Part model, mm, in its own coordinate system. Face numbers are marked on the shaded views. Give positions to 0.01 mm unless a question says otherwise; leave off trailing zeros. Order: outer loops, then holes, each group sorted by start corner. A loop starts at its lowest first (then second) coordinate and runs counter-clockwise, first axis right, second up. Notation, with made-up numbers: (12.25, 30) -> (70.25, 30) arc R22 cw to (70.25, 63) -> close; hole circle Ø5 at (65.25, -29.5). An arc over 180 degrees is marked (long way). Write item = value, one per line. Start each with the question number.
Item 1: Flat gauge pins, fed straight in: P1, Ø23, axis at x = 4, z = -10.5, coming from the -Y side; P2, Ø2, axis at x = 5.5, y = 14, coming from the +Z side; P3, Ø1, axis at y = 31, z = -0.5, coming from the -X side; P4, Ø8, axis at y = 11, z = -18, coming from the -X side. Where does each tip first touch, or does it go through?
Item 2: Band-saw the part on B-B on z = -17.5. Write the cut outline in (x, y).
Item 3: Band-saw the part on C-C on z = 20. Write the cut outline in (x, y).
Item 4: Drill centre lines: line 1 along Y through (x, z) = (1.5, -2); line 2 along X through (y, z) = (3, -0.5); line 3 along X through (y, z) = (29, 21). Where is each one in solid material? Low to high.
Item 5: Band-saw the part on A-A on y = 5. Write the cut outline in (x, z), plus the area to 3 significant figures.
Item 6: Pull direction X, two halves, no side cores. Call the marked faces 1, 2 and 3: +X half, -X half, draft (parallel to the pull), parting line (faces both ways), or undercut.
```python
from build123d import *

# Parameters (mm, degrees)
SKETCH1_R           = 22.86
BOSS_EXTRUDE1_DEPTH = 43.18
SKETCH3_R           = 3.81
BOSS_EXTRUDE2_DEPTH = 2.54
BOSS_EXTRUDE2_TAPER = 52
CIRPATTERN1_COUNT   = 8


with BuildPart() as part:
    # Sketch1 → Boss-Extrude1 (new body)
    with BuildSketch(Plane(origin=(0, 0, 0), x_dir=(1, 0, 0), z_dir=(0, 1, 0))):
        with Locations(Location((0, 0, 0), (0, 0, 270))):
            Circle(SKETCH1_R)
    extrude(amount=BOSS_EXTRUDE1_DEPTH)

    # Sketch3 → Boss-Extrude2 (add)
    with BuildSketch(Plane(origin=(0, 0, 0), x_dir=(-1, 0, 0), z_dir=(0, -1, 0))):
        with Locations((0, 11.43)):
            Circle(SKETCH3_R)
    boss_extrude2 = extrude(amount=BOSS_EXTRUDE2_DEPTH, taper=BOSS_EXTRUDE2_TAPER)

    # CirPattern1: Boss-Extrude2 ×8 about axis
    cirpattern1_axis = Axis((0, 0, 0), (0, 1, 0))
    for i in range(1, CIRPATTERN1_COUNT):
        add(boss_extrude2.rotate(cirpattern1_axis, i * 360 / CIRPATTERN1_COUNT))


solid = part.part
```
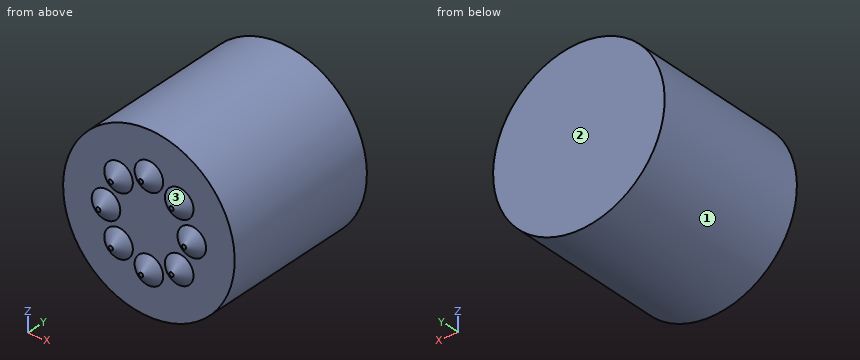
Values found:
q1.P1 = -2.54
q1.P2 = 22.41
q1.P3 = -22.86
q1.P4 = -18.07
q2.outline = (-14.71, 0) -> (14.71, 0) -> (14.71, 43.18) -> (-14.71, 43.18) -> close
q3.outline = (-11.07, 0) -> (11.07, 0) -> (11.07, 43.18) -> (-11.07, 43.18) -> close
q4.line_1 = 0 to 43.18
q4.line_2 = -22.85 to 22.85
q4.line_3 = -9.03 to 9.03
q5.outline = circle Ø45.72 at (0, 0)
q5.area = 1,640 mm^2
q6.face_1 = parting line
q6.face_2 = draft
q6.face_3 = undercut
